Read the model definition and answer for the solid it produces. Units are mm, in the model's axes. A direction names the side the tool comes from. Coordinates: 2 decimals unless noted, no trailing zeros. Order: outer loops, then holes, each group sorted by start corner. A loop starts at its lowest first (then second) coordinate and runs counter-clockwise, first axis right, second up. Notation, with made-up numbers: M 40,22 L 70,22 A22 ccw 70,30 Z; hole C -7,77 d1. An arc over 180 degrees is marked long. Use a Markdown table: item, result. Add a question column.
1) Each of these flat-tipped pins is pushed along its axis until it touches: pin 1 Ø4 at (x, z) = (-4.5, 31.5) entering from -Y; pin 2 Ø3 at (y, z) = (-10, 40) entering from -X; pin 3 Ø0.9 at (x, z) = (9, 1.5) entering from -Y. Where does it stop, or does it pass through?
2) Find section B-B on x = 0. Write down the section's boundary in (y, z), plus the area to 3 significant figures.
3) For faces 4 (the face through (0, -1, 11.04)), 5 (the face through (6.5, -4, 1)), 6 (the face through (5.827, -1.479, -1.521)), 7 (the face through (3.246, -1.479, -2.958)), determine the directions among +Z, -Z, +X, -X, +Y, -Y from which every point of the face is accessible in a straight line to the end or side of a thin tool.
4) Find section C-C on y = -1.5. Write down the section's boundary in (x, z), plus the area to 3 significant figures.
5) Find section A-A on z = 20.5. Write down the section's boundary in (x, y), plus the area to 3 significant figures.
6) The mould has two halves that part along Z. Classify faces 1 (the face through (0, -1, 31.04)), 2 (the face through (0, -1, 45.96)), 3 (the face through (0, -1, 3)): released by +Z, released by -Z, zero draft, split by the parting line, or undercut.
7) Find the intervals of material crossed by probe 1 along X at (y, z) = (-2, 15); probe 2 along Y at (x, z) = (4.25, 21.5); probe 3 along Z at (x, y) = (7, -4.25), in increasing order. Write a range as [from, to].
8) Find section D-D on z = 40. Write down the section's boundary in (x, y), plus the area to 3 significant figures.
from build123d import *

# Parameters (mm, degrees)
F0_W     = 7
F0_H     = 20
F0_R     = 3.96
F1_DEPTH = 3
F2_R     = 3.96
F3_DEPTH = 12
F4_R     = 1.25
F5_W     = 3.5
F5_H     = 3
F6_DEPTH = 2


with BuildPart() as f1:
    # F0 (on Front) → F1 (new body)
    with BuildSketch(Plane.XZ):
        Polygon((5.7, 0), (3, 0), (3.5, -6), (6.2, -6), (7, -3), (5.95, -3), align=None)
        with BuildLine():
            ThreePointArc((-3, 0), (0, 3), (3, 0))
            Line((3, 0), (5.7, 0))
            Line((5.7, 0), (10, 0))
            Line((10, 0), (10, 45.96))
            Line((10, 45.96), (-10, 45.96))
            Line((-10, 45.96), (-10, 0))
            Line((-10, 0), (-5.7, 0))
            Line((-5.7, 0), (-3, 0))
        make_face()
        with Locations((0, 21.04)):
            Rectangle(F0_W, F0_H, mode=Mode.SUBTRACT)
        with Locations((0, 40)):
            Circle(F0_R, mode=Mode.SUBTRACT)
        Polygon((-3.5, -6), (-3, 0), (-5.7, 0), (-5.95, -3), (-7, -3), (-6.2, -6), align=None)
        with Locations((0, 40)):
            Circle(F0_R)
    extrude(amount=F1_DEPTH)

    # F2 (on face) → F3 (join)
    with BuildSketch(Plane(origin=(0, 0, 0), x_dir=(-1, 0, 0), z_dir=(0, 1, 0))):
        with Locations((0, 40)):
            Circle(F2_R)
    extrude(amount=-F3_DEPTH)

    # F4
    f4_edges = [f1.edges().sort_by_distance(p)[0] for p in [
        (3.96, -12, 40),
    ]]
    fillet(f4_edges, radius=F4_R)

    # F5 (on face) → F6 (join)
    with BuildSketch(Plane.XZ.offset(3)):
        with Locations((-8.25, 1.5)):
            Rectangle(F5_W, F5_H)
        with Locations((8.25, 1.5)):
            Rectangle(F5_W, F5_H)
    extrude(amount=F6_DEPTH)


solid = f1.part
Check result:
| question | item | result |
|---|---|---|
| 1 | pin 1 | stops at y = -3 |
| 1 | pin 2 | stops at x = -3.96 |
| 1 | pin 3 | stops at y = -5 |
| 2 | outline | M -12,37.29 A1.25 ccw -10.75,36.04 L -3,36.04 L -3,31.04 L 0,31.04 L 0,45.96 L -3,45.96 L -3,43.96 L -10.75,43.96 A1.25 ccw -12,42.71 Z; M -3,3 L 0,3 L 0,11.04 L -3,11.04 Z |
| 2 | area | 139 mm2 |
| 3 | face 4 | +Y, -Y |
| 3 | face 5 | +Z, -Z, -Y |
| 3 | face 6 | +X, +Y, -Y |
| 3 | face 7 | -Z, +Y, -Y |
| 4 | outline | M -10,0 L -5.7,0 L -5.95,-3 L -7,-3 L -6.2,-6 L -3.5,-6 L -3,0 A3 cw 3,0 L 3.5,-6 L 6.2,-6 L 7,-3 L 5.95,-3 L 5.7,0 L 10,0 L 10,45.96 L -10,45.96 Z; hole M -3.5,11.04 L 3.5,11.04 L 3.5,31.04 L -3.5,31.04 Z |
| 4 | area | 801 mm2 |
| 5 | outline | M -10,-3 L -3.5,-3 L -3.5,0 L -10,0 Z; M 3.5,-3 L 10,-3 L 10,0 L 3.5,0 Z |
| 5 | area | 39.0 mm2 |
| 6 | face 1 | undercut |
| 6 | face 2 | released by +Z |
| 6 | face 3 | released by -Z |
| 7 | probe 1 | x = [-10, -3.5], [3.5, 10] |
| 7 | probe 2 | y = [-3, 0] |
| 7 | probe 3 | z = [0, 3] |
| 8 | outline | M -10,-3 L -3.96,-3 L -3.96,-10.75 A1.25 ccw -2.71,-12 L 2.71,-12 A1.25 ccw 3.96,-10.75 L 3.96,-3 L 10,-3 L 10,0 L -10,0 Z |
| 8 | area | 131 mm2 |
